Read the model definition and answer for the solid it produces. Units are mm, in the model's axes. Face numbers are marked on the shaded views. A direction names the side the tool comes from. Round coordinates to 2 decimals unless told otherwise and drop trailing zeros. Write each loop counter-clockwise with the first axis right and the second up, starting at its lowest first coordinate (ties: lowest second). Pieces come first, ordered by that corner, then holes. Notation, with made-up numbers: (-13.5, -36) - (5.5, -36) arc R20 ccw to (5.5, -7) - close; hole circle Ø7 at (73.5, 54). An arc over 180 degrees is marked (long way). Use one line per item in the form item = value. Start each with the question number.
1) The part is cut by section A-A, the plane x = 177. Give the vertices of the cut face in (y, z).
2) Each of these flat-tipped pins is pushed along its axis until it touches: pin 1 (22.5 mm diameter, centred on x = 123.5, z = 49, fed in from +Y); pin 2 (12 mm diameter, centred on y = 77.5, z = 26.5, fed in from -X); pin 3 (5 mm diameter, centred on x = 163.5, z = 35, fed in from +Y); pin 4 (9.5 mm diameter, centred on y = 72, z = 84.5, fed in from -X). Where does it stop, or does it pass through?
3) For the marked faces 1, 2 and 3, determine the directions among +Z, -Z, +X, -X, +Y, -Y from which every point of the face is accessible in a straight line to the end or side of a thin tool.
4) Consider line 1 along Z through (x, y) = (113, 71); line 2 along Z through (x, y) = (75, 67); line 3 along X through (y, z) = (55, 45). Determine where each line is inside the solid, lowest interval first. Write a range as from..to.
5) The part is cut by section D-D, the plane z = 86.5. Give the vertices of the cut face in (x, y), plus the area to 3 significant figures.
6) The part is cut by section B-B, the plane z = 70. Give the vertices of the cut face in (x, y).
7) For a pull along Z with two mould halves and no side action, classify the marked faces 4, 5 and 6 as released by +Z, released by -Z, zero draft, split by the parting line, or undercut.
from build123d import *

# Parameters (mm, degrees)
BOSS_EXTRUDE1_DEPTH = 88.89999999999999
SKETCH2_R           = 29.97200000000001
CUT_EXTRUDE1_DEPTH  = 203.2
CUT_EXTRUDE2_DEPTH  = 8.001
SKETCH4_W           = 59.943999999999946
SKETCH4_H           = 29.972
CUT_EXTRUDE3_DEPTH  = 27.94
SKETCH5_R           = 38.417500000000004
CUT_EXTRUDE4_DEPTH  = 107.696
CUT_EXTRUDE5_DEPTH  = 5.08
SKETCH7_W           = 203.19999999999996
SKETCH7_H           = 6.349999999999999
BOSS_EXTRUDE2_DEPTH = 38.1
FILLET1_R           = 2.54
CUT_EXTRUDE6_DEPTH  = 44.449999999999996


with BuildPart() as part:
    # Sketch1 → Boss-Extrude1 (new body)
    with BuildSketch(Plane(origin=(0, 0, 0), x_dir=(1, 0, 0), z_dir=(0, 1, 0))):
        Polygon((0, 0), (203.2, 0), (203.2, -101.6), (1.244e-14, -101.6), align=None)
    extrude(amount=BOSS_EXTRUDE1_DEPTH)

    # Sketch2 → Cut-Extrude1 (cut)
    with BuildSketch(Plane(origin=(203.2, 0, 0), x_dir=(-2.2e-16, 0, -1), z_dir=(1, 0, -2.2e-16))):
        with Locations((-50.8, 88.89999999999999)):
            Circle(SKETCH2_R)
    extrude(amount=-CUT_EXTRUDE1_DEPTH, mode=Mode.SUBTRACT)

    # Sketch3 → Cut-Extrude2 (cut)
    with BuildSketch(Plane(origin=(203.2, 0, 0), x_dir=(-2.2e-16, 0, -1), z_dir=(1, 0, -2.2e-16))):
        Polygon((-20.82800000000002, 118.87199999999997), (-80.77199999999996, 118.87199999999996), (-80.77199999999996, 58.928000000000004), (-20.828000000000007, 58.928000000000004), align=None)
    extrude(amount=-CUT_EXTRUDE2_DEPTH, mode=Mode.SUBTRACT)

    # Sketch4 → Cut-Extrude3 (cut)
    with BuildSketch(Plane(origin=(135.636, 0, 0), x_dir=(-2.2e-16, 0, -1), z_dir=(1, 0, -2.2e-16))):
        with Locations((-50.800000000000004, 73.914)):
            Rectangle(SKETCH4_W, SKETCH4_H)
    extrude(amount=-CUT_EXTRUDE3_DEPTH, mode=Mode.SUBTRACT)

    # Sketch5 → Cut-Extrude4 (cut)
    with BuildSketch(Plane.ZY):
        with Locations((50.8, 88.89999999999999)):
            Circle(SKETCH5_R)
    extrude(amount=-CUT_EXTRUDE4_DEPTH, mode=Mode.SUBTRACT)

    # Sketch6 → Cut-Extrude5 (cut)
    with BuildSketch(Plane(origin=(0, 58.928000000000004, 0), x_dir=(1, 0, 0), z_dir=(0, 1, 0))):
        with BuildLine():
            ThreePointArc((121.66599999999983, -34.29000000000002), (114.68100000000004, -41.275000000000006), (121.66599999999983, -48.25999999999999))
            Line((121.66600000000003, -48.25999999999999), (121.66600000000003, -34.29000000000002))
        make_face()
        with BuildLine():
            Line((121.66600000000003, -34.29000000000002), (121.66600000000003, -48.25999999999999))
            ThreePointArc((121.66599999999983, -48.25999999999999), (126.60514086658797, -46.214140866588096), (128.651, -41.275000000000006))
            ThreePointArc((128.651, -41.275000000000006), (126.60514086658797, -36.335859133411915), (121.66599999999983, -34.29000000000002))
        make_face()
    extrude(amount=-CUT_EXTRUDE5_DEPTH, mode=Mode.SUBTRACT)

    # Sketch7 → Boss-Extrude2 (add)
    with BuildSketch(Plane.XY.offset(101.6)):
        with Locations((101.59999999999998, 3.1749999999999994)):
            Rectangle(SKETCH7_W, SKETCH7_H)
    extrude(amount=BOSS_EXTRUDE2_DEPTH)

    # Fillet1
    fillet1_edges = [part.edges().sort_by_distance(p)[0] for p in [
        (101.6, 6.35, 101.6),
        (0, 6.35, 120.64999999999999),
        (203.2, 6.35, 120.64999999999999),
        (0, 44.449999999999996, 0),
        (1.168e-14, 88.89999999999999, 95.40875),
        (1.244e-14, 47.625, 101.6),
        (101.6, 88.89999999999999, 0),
        (203.2, 44.449999999999996, 0),
        (203.2, 88.89999999999999, 10.413999999999994),
        (203.2, 88.89999999999999, 91.186),
        (101.6, 88.89999999999999, 101.6),
        (203.2, 47.625, 101.6),
    ]]
    fillet(fillet1_edges, radius=FILLET1_R)

    # Sketch8 → Cut-Extrude6 (cut)
    with BuildSketch(Plane.XZ):
        Polygon((0, 139.7), (203.2, 139.7), (203.20000000000002, -1.73e-15), (1.711e-14, 0), align=None)
    extrude(amount=-CUT_EXTRUDE6_DEPTH, mode=Mode.SUBTRACT)


solid = part.part
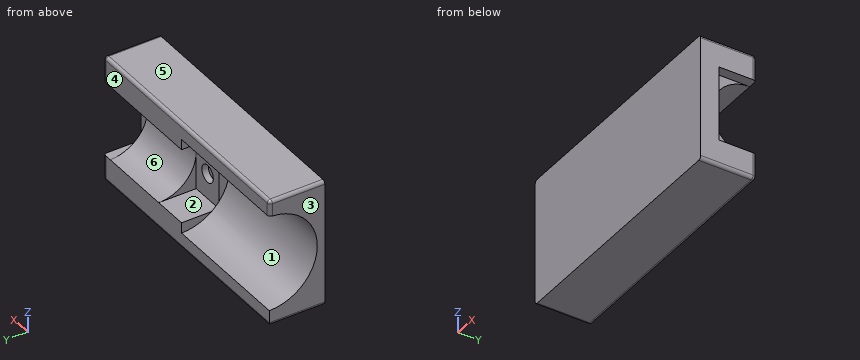
Geometry results:
q1.outline = (44.45, 0) - (86.36, 0) arc R2.54 ccw to (88.9, 2.54) - (88.9, 20.83) arc R29.97 cw to (88.9, 80.77) - (88.9, 99.06) arc R2.54 ccw to (86.36, 101.6) - (44.45, 101.6) - close
q2.pin_1 = 58.93
q2.pin_2 = 107.7
q2.pin_3 = 65.16
q2.pin_4 = 0
q3.face_1 = -X, +Y
q3.face_2 = +Y
q3.face_3 = +Z, -Z, -X, +Y, -Y
q4.line_1 = 0..20.83, 80.77..101.6
q4.line_2 = 0..19.24, 82.36..101.6
q4.line_3 = 107.7..115.76, 127.57..203.2
q5.outline = (0, 44.45) - (203.2, 44.45) - (203.2, 86.36) arc R2.54 ccw to (200.66, 88.9) - (107.7, 88.9) - (107.7, 74.71) - (0, 74.71) - close
q5.area = 7,500 mm2
q6.outline = (0, 44.45) - (203.2, 44.45) - (203.2, 58.93) - (195.2, 58.93) - (195.2, 65.89) - (135.64, 65.89) - (135.64, 58.93) - (107.7, 58.93) - (107.7, 55.62) - (0, 55.62) - close
q7.face_4 = zero draft
q7.face_5 = released by +Z
q7.face_6 = undercut
